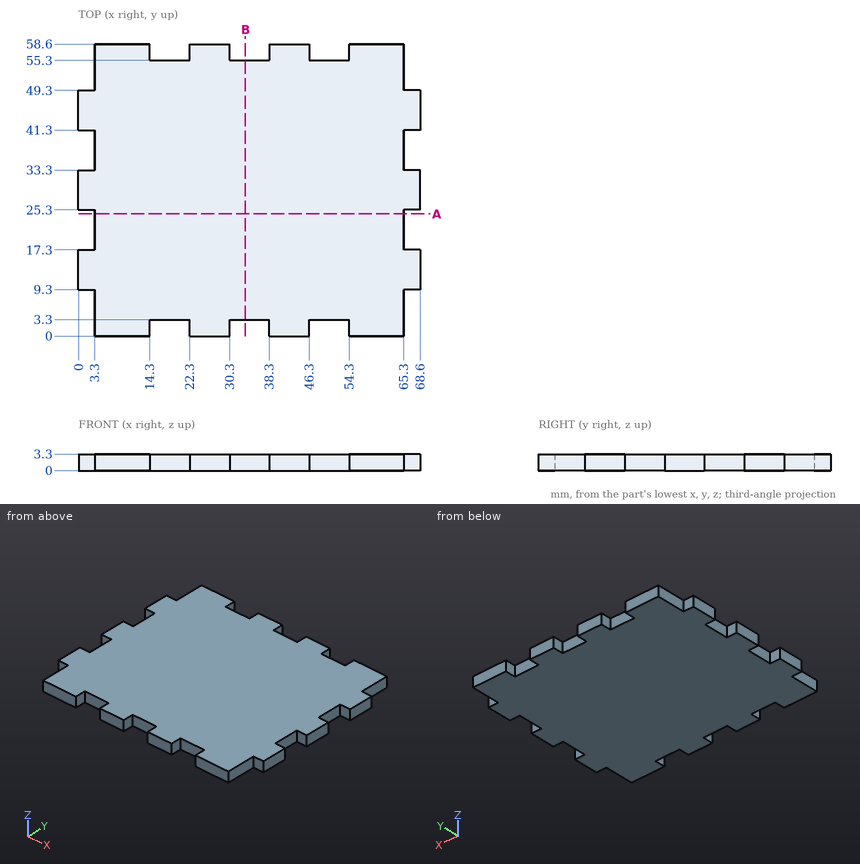
Verification items for this drawing (mm, ordinates from the low corner). Round coordinates to 2 decimals unless told otherwise and drop trailing zeros. Order: outer loops, then holes, each group sorted by start corner. A loop starts at its lowest first (then second) coordinate and runs counter-clockwise, first axis right, second up.
1) Cross-section at B-B, the plane x = 33.5. Record the cut outline in (y, z), plus the area to 3 significant figures.
Geometry says:
outline: (3.3, 0) - (55.3, 0) - (55.3, 3.3) - (3.3, 3.3) - close
area: 172 mm2
2) Depth check by flat-ended pin: pin 1 (1 mm diameter, centred on x = 52, z = 1, fed in from +Y); pin 2 (1.6 mm diameter, centred on y = 54.5, z = 2, fed in from -X); pin 3 (1 mm diameter, centred on x = 49, z = 2.5, fed in from -Y). Enter the tip coordinate at first touch or a pass-through.
Geometry says:
pin 1: stops at y = 55.3
pin 2: stops at x = 3.3
pin 3: stops at y = 3.3
3) Cross-section at A-A, the plane y = 24.5. Record the cut outline in (x, z), plus the area to 3 significant figures.
Geometry says:
outline: (3.3, 0) - (65.3, 0) - (65.3, 3.3) - (3.3, 3.3) - close
area: 205 mm2
4) Material ranges on line 1 (X direction, y = 24.5, z = 2); line 2 (Y direction, x = 49, z = 0.75), recorded low to high.
Geometry says:
line 1: x = 3.3 to 65.3
line 2: y = 3.3 to 55.3
